Work out the finished part from the listing and answer in its coordinate system (mm). A direction names the side the tool comes from. Round coordinates to 2 decimals unless told otherwise and drop trailing zeros.
1. A tool of negligible diameter and unlimited length cuts with its end or side. For faces 1 (the face through (100.013, -2, 625)), 2 (the face through (-166.018, 22.724, 630.143)), 3 (the face through (2.199, -1.788, 908.573)), from which of +Z, -Z, +X, -X, +Y, -Y can it reach the whole face along a straight path? Write none if from no direction.
2. Flat-ended cylindrical pins translate along their axes: pin 1 Ø3 at (x, y) = (-64.5, 32) entering from +Z; pin 2 Ø5 at (x, y) = (-135, 26.5) entering from -Z; pin 3 Ø2 at (x, z) = (127.5, 437) entering from -Y. Find the tip coordinate at first contact, or state that the pin passes through.
3. Straight lines are drawn through the part: probe 1 along X at (y, z) = (-13, 776.5) (1 decimal); probe 2 along X at (y, z) = (10, 761); probe 3 along Y at (x, z) = (40, 921.5). For each, find the intervals that lie inside material, in ascending order.
4. Determine the mould class of faces 4 (the face through (100.35, 81.58, 403.7)), 5 (the face through (85.725, -14, 630)), 6 (the face through (-171.45, 74, 625)) for opening direction X: pulls with the +X half, pulls with the -X half, needs draft (parallel to the pull), parting line crosses it, or undercut.
```python
from build123d import *

# Parameters (mm, degrees)
BOSS_EXTRUDE1_DEPTH           = 152.4
FILLET1_R                     = 25.4
BOSS_EXTRUDE2_DEPTH           = 50.8
BOSS_EXTRUDE3_DEPTH           = 25.4
FILLET2_R                     = 25.4
SKETCH5_W                     = 63.5
SKETCH5_H                     = 50.8
BOSS_EXTRUDE4_DEPTH           = 76.2
BOSS_EXTRUDE4_DRAFT           = 5
BOSS_EXTRUDE4_PROFILE_2_DEPTH = 76.2
BOSS_EXTRUDE4_PROFILE_2_DRAFT = 5
FILLET3_R                     = 12.7
SKETCH7_RX                    = 12.7
SKETCH7_RY                    = 12.651672666
CUT_EXTRUDE2_DEPTH            = 1182.416868754
SCALE1_SCALE                  = 0.75


with BuildPart() as part:
    # Sketch1 → Boss-Extrude1 (new body)
    with BuildSketch(Plane(origin=(0, 0, 0), x_dir=(1, 0, 0), z_dir=(0, 1, 0))):
        with BuildLine():
            Line((228.6, -342.051110312), (-228.6, -342.051110312))
            Line((-228.6, -342.051110312), (-228.6, -850.051110312))
            ThreePointArc((-228.6, -850.051110312), (0, -1078.651110312), (228.6, -850.051110312))
            Line((228.6, -850.051110312), (228.6, -342.051110312))
        make_face()
    extrude(amount=BOSS_EXTRUDE1_DEPTH)

    # Fillet1
    fillet1_edges = [part.edges().sort_by_distance(p)[0] for p in [
        (-228.6, 152.4, 596.051110312),
        (0, 152.4, 1078.651110312),
        (228.6, 152.4, 596.051110312),
        (0, 152.4, 342.051110312),
        (228.6, 0, 596.051110312),
        (0, 0, 1078.651110312),
        (-228.6, 0, 596.051110312),
        (0, 0, 342.051110312),
        (228.6, 76.2, 342.051110312),
        (-228.6, 76.2, 342.051110312),
    ]]
    fillet(fillet1_edges, radius=FILLET1_R)

    # Sketch3 → Boss-Extrude2 (add)
    with BuildSketch(Plane.XZ):
        with BuildLine():
            Line((-133.35, 850.051110312), (-133.35, 367.451110312))
            Line((-133.35, 367.451110312), (-114.3, 367.451110312))
            Line((-114.3, 367.451110312), (-114.3, 850.051110312))
            ThreePointArc((-114.3, 850.051110312), (0, 964.351110312), (114.3, 850.051110312))
            Line((114.3, 850.051110312), (114.3, 367.451110312))
            Line((114.3, 367.451110312), (133.35, 367.451110312))
            Line((133.35, 367.451110312), (133.35, 850.051110312))
            ThreePointArc((133.35, 850.051110312), (0, 983.401110312), (-133.35, 850.051110312))
        make_face()
    extrude(amount=BOSS_EXTRUDE2_DEPTH)

    # Sketch4 → Boss-Extrude3 (add)
    with BuildSketch(Plane.XZ):
        with BuildLine():
            Line((-114.3, 850.051110312), (-114.3, 367.451110312))
            Line((-114.3, 367.451110312), (114.3, 367.451110312))
            Line((114.3, 367.451110312), (114.3, 850.051110312))
            ThreePointArc((114.3, 850.051110312), (0, 964.351110312), (-114.3, 850.051110312))
        make_face()
    extrude(amount=BOSS_EXTRUDE3_DEPTH)

    # Fillet2
    fillet2_edges = [part.edges().sort_by_distance(p)[0] for p in [
        (123.825, -50.8, 367.451110312),
        (-123.825, -50.8, 367.451110312),
        (0, -25.4, 367.451110312),
    ]]
    fillet(fillet2_edges, radius=FILLET2_R - 0.0001)  # a hair under: the kernel refuses the full size


with BuildPart() as boss_extrude4_tool:
    # Sketch5 → Boss-Extrude4 (with draft: the straight prism first)
    with BuildSketch(Plane(origin=(0, 0, 342.051110312), x_dir=(-1, 0, 0), z_dir=(0, 0, -1))):
        with Locations((133.35, 63.5)):
            Rectangle(SKETCH5_W, SKETCH5_H)
    extrude(amount=BOSS_EXTRUDE4_DEPTH)
    # Boss-Extrude4: the draft: its side faces are tilted about the plane it starts from
    boss_extrude4_sides = [boss_extrude4_tool.faces().sort_by_distance(p)[0] for p in [
        (-101.6, 63.5, 303.951110312),
        (-133.35, 38.1, 303.951110312),
        (-165.1, 63.5, 303.951110312),
        (-133.35, 88.9, 303.951110312),
    ]]
    draft(boss_extrude4_sides, Plane(origin=(0, 0, 342.051110312), x_dir=(-1, 0, 0), z_dir=(0, 0, -1)), BOSS_EXTRUDE4_DRAFT)


with BuildPart() as part_1:
    add(part.part)

    # Boss-Extrude4: add boss_extrude4_tool
    add(boss_extrude4_tool.part)


with BuildPart() as boss_extrude4_profile_2_tool:
    # Sketch5 → Boss-Extrude4 profile 2 (with draft: the straight prism first)
    with BuildSketch(Plane(origin=(0, 0, 342.051110312), x_dir=(-1, 0, 0), z_dir=(0, 0, -1))):
        with Locations((-133.35, 63.5)):
            Rectangle(SKETCH5_W, SKETCH5_H)
    extrude(amount=BOSS_EXTRUDE4_PROFILE_2_DEPTH)
    # Boss-Extrude4 profile 2: the draft: its side faces are tilted about the plane it starts from
    boss_extrude4_profile_2_sides = [boss_extrude4_profile_2_tool.faces().sort_by_distance(p)[0] for p in [
        (101.6, 63.5, 303.951110312),
        (133.35, 88.9, 303.951110312),
        (165.1, 63.5, 303.951110312),
        (133.35, 38.1, 303.951110312),
    ]]
    draft(boss_extrude4_profile_2_sides, Plane(origin=(0, 0, 342.051110312), x_dir=(-1, 0, 0), z_dir=(0, 0, -1)), BOSS_EXTRUDE4_PROFILE_2_DRAFT)


with BuildPart() as part_2:
    add(part_1.part)

    # Boss-Extrude4 profile 2: add boss_extrude4_profile_2_tool
    add(boss_extrude4_profile_2_tool.part)

    # Fillet3
    fillet3_edges = [part_2.edges().sort_by_distance(p)[0] for p in [
        (133.35, 82.233363839, 265.851110312),
        (133.35, 44.766636161, 265.851110312),
        (-133.35, 44.766636161, 265.851110312),
        (-133.35, 82.233363839, 265.851110312),
    ]]
    fillet(fillet3_edges, radius=FILLET3_R)

    # Sketch7 → Cut-Extrude2 (cut, through all)
    with BuildSketch(Plane.ZY.offset(228.6)):
        with Locations(Location((288.946136063, 63.5), (0, 0, 90))):
            Ellipse(SKETCH7_RX, SKETCH7_RY)
    extrude(amount=-CUT_EXTRUDE2_DEPTH, mode=Mode.SUBTRACT)


with BuildPart() as part_3:
    # Scale1: scaled about (1.9e-07, 67.979865598, 684.18432939)
    add(part_2.part.scale(SCALE1_SCALE).moved(Location((4.8e-08, 16.9949664, 171.046082348))))


solid = part_3.part
```
Worked answers:
1. face 1: +Z, -Z, +X, -Y
1. face 2: +Z, -Z, -X, -Y
1. face 3: +Z, -Y
2. pin 1: stops at z = 967.65
2. pin 2: stops at z = 428.93
2. pin 3: stops at y = 19.06
3. probe 1: x = -100 to -85.7, 85.7 to 100
3. probe 2: x = -100.01 to 100.01
3. probe 3: y = 16.99 to 131.29
4. face 4: needs draft
4. face 5: undercut
4. face 6: pulls with the -X half
